Verification items for the finished model (mm, model axes). A direction names the side the tool comes from. Coordinates: 2 decimals unless noted, no trailing zeros. Write each loop counter-clockwise with the first axis right and the second up, starting at its lowest first coordinate (ties: lowest second). Pieces come first, ordered by that corner, then holes. Notation, with made-up numbers: (11, 19.5) -> (68, 19.5) arc R12 ccw to (68, 23.5) -> close; hole circle Ø4 at (-25, -4.5). An arc over 180 degrees is marked (long way). Use a Markdown table: item, result. Add a question column.
Autodesk Inventor part; units mm, degrees
ref_plane "YZ Plane" through (0, 0, 0) normal (1, 0, 0) x (0, 1, 0)
ref_plane "XZ Plane" through (0, 0, 0) normal (0, 1, 0) x (-1, 0, 0)
ref_plane "XY Plane" through (0, 0, 0) normal (0, 0, 1) x (1, 0, 0)
sketch "Sketch1" plane through (0, 0, 0) normal (0, 0, 1) x (1, 0, 0)
  line L0 (0, 0) -> (-50, 0)
  line L1 (-50, 40) -> (0, 40)
  line L2 (0, 40) -> (0, 0)
  line L3 (-50, 0) -> (-50, 40)
  line L4 (-50, 0) -> (-5, 0)
  line L5 (-5, 0) -> (-5, -5)
  line L6 (-5, -5) -> (-50, -5)
  line L7 (-50, -5) -> (-50, 0)
  dimension "d1" = 40
  dimension "d2" = 50
  dimension "d20" = 5
  dimension "d21" = 5
extrude "Extrusion1" add sketch "Sketch1" along normal blind 10
sketch "Sketch2" plane through (0, 0, 10) normal (0, 0, 1) x (1, 0, 0)
  line L0 (0, 40) -> (-50, 40)
  line L1 (0, 0) -> (0, 40)
  line L2 (-5, 0) -> (0, 0)
  line L3 (-50, 40) -> (-50, -5)
  point P0 (-42.5, 32.5)
  point P1 (-7.5, 7.5)
  point P2 (-50, 0)
  dimension "d5" = 7.5
  dimension "d7" = 7.5
  dimension "d15" = 7.5
  dimension "d16" = 7.5
hole "Hole1" at (-42.5, 32.5, 10) at (-7.5, 7.5, 10) direction (0, 0, -1) diameter 4.5 end through all countersink diameter 9.4 countersink angle 90
chamfer "Chamfer1" distance 30 angle 55 1 edges at (0, 40, 5) measured on face at (0, 26.6667, 3.3333)
fillet "Fillet1" radius 2 1 edges at (-5, 0, 5)
sketch "Sketch3" plane through (0, 0, 10) normal (0, 0, 1) x (1, 0, 0)
  line L0 (-50, -5) -> (-5, -5)
  line L1 (0, 0) -> (0, 10)
  point P0 (-15, 0)
  dimension "d23" = 5
  dimension "d24" = 15
hole "Hole2" at (-15, 0, 10) direction (0, 0, -1) diameter 1.694 depth 6.637 tip angle 118
properties part number "Pancake_Side Piece Short" material "Wood (Birch)"
1) Cross-section at A-A on z = 4. Record the boundary of the cut face in (x, y), then the cut area to 3 significant figures.
2) Cross-section at C-C on x = -7.5. Record the boundary of the cut face in (y, z).
3) Thickness scan on L1, parallel to X at y = 7.5, z = 4.25; L2, parallel to Y at x = -15, z = 5; L3, parallel to X at y = 32.5, z = 3.25. Record the ranges inside material, lowest first.
4) Cross-section at B-B on y = 7.5. Record the boundary of the cut face in (x, z), then the cut area to 3 significant figures.
5) Release check for a two-part mould opening along X. For faces 1 (the face through (-31, 13, 0)), 2 (the face through (-9.63, 6.39, 7.7)), 3 (the face through (-44.397, 31.29, 3.722)), 4 (the face through (0, 5, 5)) record: released by +X, released by -X, zero draft, split by the parting line, or undercut.
6) Cross-section at D-D on x = -27. Record the boundary of the cut face in (y, z).
7) Set-up check for faces 5 (the face through (-5, -3, 5)), 6 (the face through (-21.72, 25.21, 5.07)), 7 (the face through (-14.173, 0.184, 6.635)): record each of +Z, -Z, +X, -X, +Y, -Y from which the full face is reachable in a straight line by a thin tool's end or side.
8) Gauge pin test, flat ends, axial feed: pin 1 (0.9 mm diameter, centred on y = -3.5, z = 3, fed in from +X); pin 2 (3.5 mm diameter, centred on x = -2, z = 3.5, fed in from -Y). Record the tip position at first contact, or that the pin passes through.
Returned:
| question | item | result |
|---|---|---|
| 1 | outline | (-50, -5) -> (-5, -5) -> (-5, -2) arc R2 cw to (-3, 0) -> (0, 0) -> (0, 10) -> (-42.84, 40) -> (-50, 40) -> close; hole circle Ø4.5 at (-42.5, 32.5); hole circle Ø1.69 at (-15, 0); hole circle Ø4.5 at (-7.5, 7.5) |
| 1 | area | 1,550 mm² |
| 2 | outline | (-5, 0) -> (5.25, 0) -> (5.25, 7.55) -> (2.8, 10) -> (-5, 10) -> close; (9.75, 0) -> (15.25, 0) -> (15.25, 10) -> (12.2, 10) -> (9.75, 7.55) -> close |
| 3 | L1 | x = -50 to -9.75, -5.25 to 0 |
| 3 | L2 | y = -5 to -0.85, 0.85 to 20.5 |
| 3 | L3 | x = -50 to -44.75, -40.25 to -32.13 |
| 4 | outline | (-50, 0) -> (-9.75, 0) -> (-9.75, 7.55) -> (-12.2, 10) -> (-50, 10) -> close; (-5.25, 0) -> (0, 0) -> (0, 10) -> (-2.8, 10) -> (-5.25, 7.55) -> close |
| 4 | area | 449 mm² |
| 5 | face 1 | zero draft |
| 5 | face 2 | undercut |
| 5 | face 3 | undercut |
| 5 | face 4 | released by +X |
| 6 | outline | (-5, 0) -> (28.91, 0) -> (28.91, 10) -> (-5, 10) -> close |
| 7 | face 5 | +Z, -Z, +X, -Y |
| 7 | face 6 | +Z, -Z, +X, +Y |
| 7 | face 7 | +Z |
| 8 | pin 1 | stops at x = -5 |
| 8 | pin 2 | stops at y = -0.15 |
